Part model, mm, in its own coordinate system. Face numbers are marked on the shaded views. A direction names the side the tool comes from. Give positions to 0.01 mm unless a question says otherwise; leave off trailing zeros. Order: outer loops, then holes, each group sorted by start corner. A loop starts at its lowest first (then second) coordinate and runs counter-clockwise, first axis right, second up.
1. Slice it at A-A on y = 0. List the corners of the cut face in (x, z), and give its area (3 significant figures).
2. Which spindle directions (+Z, -Z, +X, -X, +Y, -Y) get a long thin tool onto all of the face, cutting with end or side? Do the marked faces 5 and 6. Say none if no direction does.
3. Probe line 1 (Y direction, x = 0, z = 27); line 2 (Y direction, x = 0, z = 7); line 3 (Y direction, x = 0, z = 1). List the from-to ranges inside material, lowest first.
4. Mould opens along X. For the marked faces 1, 2, 3 and 4 say: +X half, -X half, draft (parallel to the pull), parting line (faces both ways), or undercut.
5. Slice it at D-D on x = 0. Give the number of separate pieces and of enclosed holes in the cut face, and give its area (3 significant figures).
6. Slice it at C-C on z = 25. List the corners of the cut face in (x, y).
7. Drop flat-ended pins along their axis: pin 1 Ø1 at (y, z) = (7.5, 26) entering from -X; pin 2 Ø1 at (x, y) = (-10.5, -11.5) entering from +Z; pin 3 Ø4 at (y, z) = (-2.5, 19) entering from -X; pin 4 Ø4 at (x, z) = (0, 25) entering from -Y. Give the stop position or say it passes through.
8. Slice it at B-B on z = 35.5. List the corners of the cut face in (x, y), and give its area (3 significant figures).
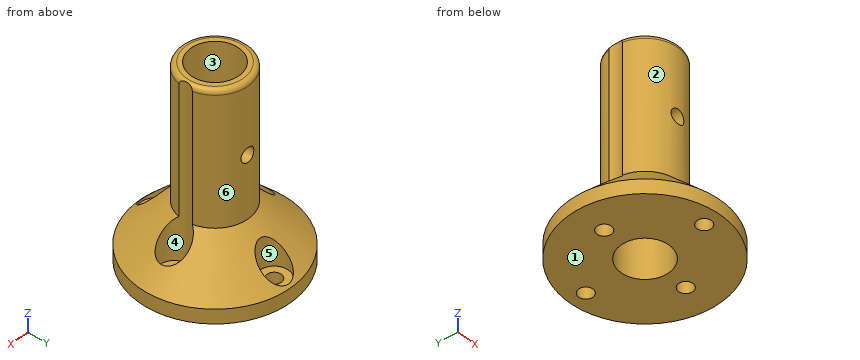
from build123d import *

# Parameters (mm, degrees)
SKETCH_1_R               = 16
EXTRUDE_1_DEPTH          = 40
SKETCH_2_W               = 5.07
SKETCH_2_H               = 40
SKETCH_3_R               = 1.5
CUT_EXTRUDE_2_DEPTH      = 46.956501172
SKETCH_4_R               = 3
SKETCH_4_R_2             = 1.5
CUT_EXTRUDE_3_DEPTH      = 44.370496958
CUT_EXTRUDE_4_DEPTH      = 46.956501329
CUT_EXTRUDE_4_DEPTH_BACK = 46.956501329
SKETCH_5_R               = 1.5


with BuildPart() as part:
    # 草图1 → 凸台-拉伸1 (new body)
    with BuildSketch(Plane.XY):
        Circle(SKETCH_1_R)
    extrude(amount=EXTRUDE_1_DEPTH)

    # 草图2 → 切除-旋转1 (revolve, cut)
    with BuildSketch(Plane(origin=(0, 0, 0), x_dir=(1, 0, 0), z_dir=(0, 1, 0))):
        Polygon((-16, -40), (-16, -3), (-7, -12), (-7, -40), align=None)
        with Locations((-2.535, -20)):
            Rectangle(SKETCH_2_W, SKETCH_2_H)
    revolve(axis=Axis((0, 0, 0), (0, 0, 1)), mode=Mode.SUBTRACT)

    # 草图3 → 切除-拉伸2 (cut, through all)
    with BuildSketch(Plane.XY):
        with Locations(Location((0, -12.5, 0), (0, 0, 237.240983175))):
            Circle(SKETCH_3_R)
        with Locations(Location((-9.5, 0, 0), (0, 0, 179.999999805))):
            Circle(SKETCH_3_R)
        with Locations(Location((9.5, 0, 0), (0, 0, 259.790179824))):
            Circle(SKETCH_3_R)
        with Locations(Location((0, 12.5, 0), (0, 0, 122.759016825))):
            Circle(SKETCH_3_R)
    extrude(amount=CUT_EXTRUDE_2_DEPTH, mode=Mode.SUBTRACT)

    # 草图4 → 切除-拉伸3 (cut, through all)
    # profile 1 of 4: a face of its own
    with BuildSketch(Plane.XY.offset(3)):
        with Locations(Location((0, 12.5, 0), (0, 0, 206.851583032))):
            Circle(SKETCH_4_R)
        with Locations((0, 12.5)):
            Circle(SKETCH_4_R_2, mode=Mode.SUBTRACT)
    # profile 2 of 4: a face of its own
    with BuildSketch(Plane.XY.offset(3)):
        with Locations(Location((-9.5, 0, 0), (0, 0, 179.999999996))):
            Circle(SKETCH_4_R)
        with Locations((-9.5, 0)):
            Circle(SKETCH_4_R_2, mode=Mode.SUBTRACT)
    # profile 3 of 4: a face of its own
    with BuildSketch(Plane.XY.offset(3)):
        with Locations(Location((9.5, 0, 0), (0, 0, 208.166578237))):
            Circle(SKETCH_4_R)
        with Locations((9.5, 0)):
            Circle(SKETCH_4_R_2, mode=Mode.SUBTRACT)
    # profile 4 of 4: a face of its own
    with BuildSketch(Plane.XY.offset(3)):
        with Locations(Location((0, -12.5, 0), (0, 0, 225.843438768))):
            Circle(SKETCH_4_R)
        with Locations((0, -12.5)):
            Circle(SKETCH_4_R_2, mode=Mode.SUBTRACT)
    extrude(amount=CUT_EXTRUDE_3_DEPTH, mode=Mode.SUBTRACT)

    # 草图5 → 切除-拉伸4 (cut, two sides: drawn at the far end of the back side and taken through both)
    with BuildSketch(Plane(origin=(0, 0, 0), x_dir=(1, 0, 0), z_dir=(0, 1, 0)).offset(-CUT_EXTRUDE_4_DEPTH_BACK)):
        with Locations(Location((0, -25, 0), (0, 0, 270))):
            Circle(SKETCH_5_R)
    extrude(amount=CUT_EXTRUDE_4_DEPTH + CUT_EXTRUDE_4_DEPTH_BACK, mode=Mode.SUBTRACT)

    # 圆角1: read off the stored shape, not the designer's step
    # 圆角1 outline → 圆角1 (revolve, cut)
    with BuildSketch(Plane.XZ):
        with BuildLine():
            ThreePointArc((6, 40), (6.707106781, 39.707106781), (7, 39))
            Line((7, 39), (7, 40))
            Line((7, 40), (6, 40))
        make_face()
    revolve(axis=Axis((0, 0, 0), (0, 0, 1)), mode=Mode.SUBTRACT)


solid = part.part
Data:
1. outline: (-16, 0) - (-11, 0) - (-11, 3) - (-12.5, 3) - (-12.5, 6.5) - (-16, 3) - close; (-8, 0) - (-5.07, 0) - (-5.07, 40) - (-6, 40) arc R1 ccw to (-6.5, 39.87) - (-6.5, 3) - (-8, 3) - close; (5.07, 0) - (8, 0) - (8, 3) - (6.5, 3) - (6.5, 39.87) arc R1 ccw to (6, 40) - (5.07, 40) - close; (11, 0) - (16, 0) - (16, 3) - (12.5, 6.5) - (12.5, 3) - (11, 3) - close
1. area: 166 mm2
2. face 5: +Z
2. face 6: +Z, +Y
3. line 1: y = -7 to -5.07, 5.07 to 7
3. line 2: y = -9.5 to -5.07, 5.07 to 9.5
3. line 3: y = -16 to -14, -11 to -5.07, 5.07 to 11, 14 to 16
4. face 1: draft
4. face 2: parting line
4. face 3: undercut
4. face 4: undercut
5. separate pieces: 6
5. enclosed holes: 0
5. area: 217 mm2
6. outline: (-6.86, -1.42) arc R7 ccw to (-1.5, -6.84) - (-1.5, -4.84) arc R5.07 cw to (-1.5, 4.84) - (-1.5, 6.84) arc R7 ccw to (-6.86, 1.42) arc R3 cw to start; (1.5, -6.84) arc R7 ccw to (6.86, -1.42) arc R3 cw to (6.86, 1.42) arc R7 ccw to (1.5, 6.84) - (1.5, 4.84) arc R5.07 cw to (1.5, -4.84) - close
7. pin 1: passes through
7. pin 2: stops at z = 3.93
7. pin 3: stops at x = -6.86
7. pin 4: stops at y = -7
8. outline: (-6.86, -1.42) arc R7 ccw to (6.86, -1.42) arc R3 cw to (6.86, 1.42) arc R7 ccw to (-6.86, 1.42) arc R3 cw to start; hole circle Ø10.14 at (0, 0)
8. area: 71.3 mm2
